```python
from build123d import *

# Parameters (mm, degrees)
SKETCH1_R           = 7
SKETCH1_R_2         = 14
BOSS_EXTRUDE1_DEPTH = 12
FILLET1_R           = 50


with BuildPart() as part:
    # Sketch1 → Boss-Extrude1 (new body)
    with BuildSketch(Plane.XY):
        with BuildLine():
            Line((-18.395196505, 48.755706629), (-31, 0))
            Line((-31, 0), (-18.395196505, -48.755706629))
            ThreePointArc((-18.395196505, -48.755706629), (0, -63), (18.395196505, -48.755706629))
            Line((18.395196505, -48.755706629), (31, 0))
            Line((31, 0), (18.395196505, 48.755706629))
            ThreePointArc((18.395196505, 48.755706629), (0, 63), (-18.395196505, 48.755706629))
        make_face()
        with Locations((0, 44)):
            Circle(SKETCH1_R, mode=Mode.SUBTRACT)
        with Locations((0, -44)):
            Circle(SKETCH1_R, mode=Mode.SUBTRACT)
        Circle(SKETCH1_R_2, mode=Mode.SUBTRACT)
    extrude(amount=BOSS_EXTRUDE1_DEPTH)

    # Fillet1
    fillet1_edges = [part.edges().sort_by_distance(p)[0] for p in [
        (31, 0, 6),
        (-31, 0, 6),
    ]]
    fillet(fillet1_edges, radius=FILLET1_R)

    # Sketch3 → Revolve1 (revolve)
    with BuildSketch(Plane(origin=(0, 0, 0), x_dir=(1, 0, 0), z_dir=(0, 1, 0)), mode=Mode.PRIVATE) as revolve1_sk:
        Polygon((14, -12), (28, -12), (28, -42), (14, -33.917096231), align=None)
    revolve(revolve1_sk.sketch.rotate(Axis((0, 0, -17.419804193), (0, 0, 1)), 180), axis=Axis((0, 0, -17.419804193), (0, 0, 1)))


solid = part.part
```
Verification items for the finished model (mm, model axes). A direction names the side the tool comes from. Give positions to 0.01 mm unless a question says otherwise; leave off trailing zeros. Order: outer loops, then holes, each group sorted by start corner. A loop starts at its lowest first (then second) coordinate and runs counter-clockwise, first axis right, second up. Notation, with made-up numbers: M 79,-31 L 99,-31 A22 cw 99,-6 Z; hole C -11,82 d9. An arc over 180 degrees is marked long. Answer in a Markdown table with one row per item. Add a question column.
Item 1: Section check D-D, the plane y = 29.5. Enter the section's corners in (x, z), and give its area (3 significant figures).
Item 2: Section check C-C, the plane z = 21.5. Enter the section's corners in (x, y), and give its area (3 significant figures).
Item 3: Mould release check, pull along X, two halves, no side actions. Record for faces 3 (the flat face through (-23.145, -30.382, 5.916)), 4 (the flat face through (23.014, -30.889, 5.916)), 5 (the conical face through (3.18, 14.33, 34.31)), 6 (the cylindrical face through (0, -63, 6)): released by +X, released by -X, zero draft, split by the parting line, or undercut.
Item 4: Gauge pin test, flat ends, axial feed: pin 1 (5 mm diameter, centred on x = 21.5, z = 36, fed in from -Y); pin 2 (1 mm diameter, centred on x = -8, z = 30, fed in from -Y); pin 3 (6 mm diameter, centred on y = -39, z = 14.5, fed in from +X); pin 4 (17 mm diameter, centred on x = 0, y = 0, fed in from +Z). Record the tip position at first contact, or that the pin passes through.
Item 5: Section check B-B, the plane y = -44. Enter the section's corners in (x, z), and give its area (3 significant figures).
Item 6: Tool access check on faces 1 (the cylindrical face through (-25.865, 10.724, 27.21)), 2 (the flat face through (23.145, 30.382, 5.916)). Record the directions out of +Z, -Z, +X, -X, +Y, -Y that give a thin tool (end or side, any length) a straight path to the whole face; none if there is none.
Item 7: Scan lines: probe 1 along Y at (x, z) = (0, 13); probe 2 along Z at (x, y) = (-2, -51); probe 3 along X at (y, z) = (-10, 6.5). Record each from-to range of solid material in increasing order. Write a range as from..to.
Filled sheet:
| question | item | result |
|---|---|---|
| 1 | outline | M -23.37,0 L 23.37,0 L 23.37,12 L -23.37,12 Z |
| 1 | area | 561 mm^2 |
| 2 | outline | C 0,0 d56; hole C 0,0 d28 |
| 2 | area | 1,850 mm^2 |
| 3 | face 3 | released by -X |
| 3 | face 4 | released by +X |
| 3 | face 5 | undercut |
| 3 | face 6 | split by the parting line |
| 4 | pin 1 | stops at y = -20.57 |
| 4 | pin 2 | stops at y = -26.98 |
| 4 | pin 3 | stops at x = 21.35 |
| 4 | pin 4 | passes through |
| 5 | outline | M -19.62,0 L -7,0 L -7,12 L -19.62,12 Z; M 7,0 L 19.62,0 L 19.62,12 L 7,12 Z |
| 5 | area | 303 mm^2 |
| 6 | face 1 | +Z |
| 6 | face 2 | +Z, -Z, +X, +Y |
| 7 | probe 1 | y = -28..-14, 14..28 |
| 7 | probe 2 | z = 0..12 |
| 7 | probe 3 | x = -28.35..-9.8, 9.8..28.35 |
